```python
from build123d import *

# Parameters (mm, degrees)
SKETCH1_W           = 53.98
SKETCH1_H           = 1.59
SKETCH1_W_2         = 6.35
BOSS_EXTRUDE1_DEPTH = 20.64
SKETCH1_3_W         = 53.98
SKETCH1_3_H         = 1.59
SKETCH1_3_H_2       = 18.25
SKETCH1_3_R         = 3.175
SKETCH1_3_W_2       = 6.35
SKETCH1_3_H_3       = 19.84
BOSS_EXTRUDE2_DEPTH = 1.59


with BuildPart() as part:
    # Sketch1 → Boss-Extrude1 (new body)
    with BuildSketch(Plane(origin=(0, 0, 0), x_dir=(1, 0, 0), z_dir=(0, 1, 0))):
        with Locations((0, 0.005)):
            Rectangle(SKETCH1_W, SKETCH1_H)
        with Locations((-30.165, 0.005)):
            Rectangle(SKETCH1_W_2, SKETCH1_H)
        with Locations((30.165, 0.005)):
            Rectangle(SKETCH1_W_2, SKETCH1_H)
    extrude(amount=BOSS_EXTRUDE1_DEPTH)

    # Sketch1_3 → Boss-Extrude2 (add)
    # profile 1 of 4: a face of its own
    with BuildSketch(Plane(origin=(0, 0, 0), x_dir=(1, 0, 0), z_dir=(0, 1, 0))):
        with Locations((0, 0.005)):
            Rectangle(SKETCH1_3_W, SKETCH1_3_H)
    # profile 2 of 4: a face of its own
    with BuildSketch(Plane(origin=(0, 0, 0), x_dir=(1, 0, 0), z_dir=(0, 1, 0))):
        with Locations((0, 9.925)):
            Rectangle(SKETCH1_3_W, SKETCH1_3_H_2)
        with Locations(Location((-13.825, 10.08, 0), (0, 0, 90))):
            Circle(SKETCH1_3_R, mode=Mode.SUBTRACT)
        with Locations(Location((13.825, 10.08, 0), (0, 0, 90))):
            Circle(SKETCH1_3_R, mode=Mode.SUBTRACT)
    # profile 3 of 4: a face of its own
    with BuildSketch(Plane(origin=(0, 0, 0), x_dir=(1, 0, 0), z_dir=(0, 1, 0))):
        with Locations((-30.165, 9.13)):
            Rectangle(SKETCH1_3_W_2, SKETCH1_3_H_3)
    # profile 4 of 4: a face of its own
    with BuildSketch(Plane(origin=(0, 0, 0), x_dir=(1, 0, 0), z_dir=(0, 1, 0))):
        with Locations((30.165, 9.13)):
            Rectangle(SKETCH1_3_W_2, SKETCH1_3_H_3)
    extrude(amount=BOSS_EXTRUDE2_DEPTH)


solid = part.part
```
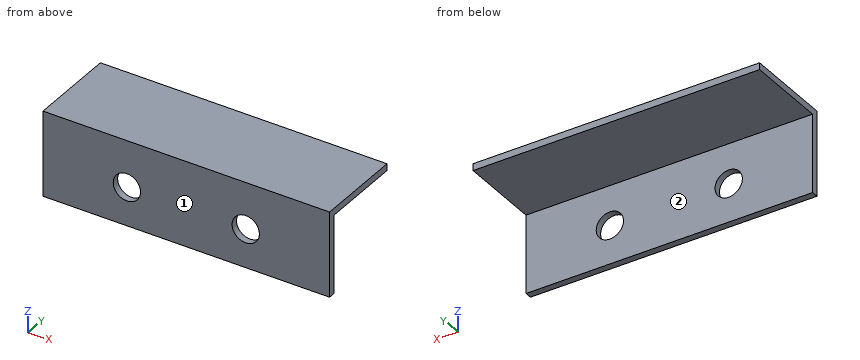
Can you work these out from the model? Positions are in its coordinate system, mm. Face numbers are marked on the shaded views. A direction names the side the tool comes from. Coordinates: 2 decimals unless noted, no trailing zeros. Write each loop counter-clockwise with the first axis right and the second up, starting at its lowest first coordinate (ties: lowest second). Pieces come first, ordered by that corner, then holes. Notation, with made-up numbers: M 56,-1.5 L 90,-1.5 A22 ccw 90,14.5 Z; hole C -14.75,71 d9. An arc over 180 degrees is marked long. Write item = value, one per line. Start each with the question number.
Q1. If we section it at B-B, the plane x = 24: Write out the boundary of the cut face in (y, z).
Q2. If we section it at C-C, the plane z = -16.75: Write out the boundary of the cut face in (x, y).
Q3. I'm going to push flat-ended pins straight in: pin 1 (4 mm diameter, centred on x = -2.5, y = 16, fed in from -Z); pin 2 (5 mm diameter, centred on x = 16.5, z = -4.5, fed in from +Y); pin 3 (4 mm diameter, centred on x = 13.825, z = -10.08, fed in from -Y). Where does each tip first touch, or does it pass through?
Q4. If we section it at D-D, the plane y = 2.5: Write out the boundary of the cut face in (x, z), then the cut area to 3 significant figures.
Q5. If I drill on L1, parallel to X at y = 0.3, z = -10.08; L2, parallel to Y at x = 24, z = -14.75; L3, parallel to Z at x = 28.5, y = 5, over which ranges is the centre line in solid material (lowest first)? Write a range as [from, to].
Q6. If we section it at A-A, the plane z = -10.08: Write out the boundary of the cut face in (x, y).
Q7. On a 3-axis mill with a long thin cutter (end or side, diameter ignored), from which of +Z, -Z, +X, -X, +Y, -Y can I reach the whole of each face in a straight line? I mean the marked faces 1 and 2. Say none if no direction works.
Check sheet entries:
q1.outline = M 0,-19.05 L 1.59,-19.05 L 1.59,-0.8 L 20.64,-0.8 L 20.64,0.79 L 0,0.79 Z
q2.outline = M -33.34,0 L 33.34,0 L 33.34,1.59 L -33.34,1.59 Z
q3.pin_1 = -0.8
q3.pin_2 = 1.59
q3.pin_3 = through
q4.outline = M -33.34,-0.8 L 33.34,-0.8 L 33.34,0.79 L -33.34,0.79 Z
q4.area = 106 mm²
q5.L1 = [-33.34, -17], [-10.65, 10.65], [17, 33.34]
q5.L2 = [0, 1.59]
q5.L3 = [-0.8, 0.79]
q6.outline = M -33.34,0 L -17,0 L -17,1.59 L -33.34,1.59 Z; M -10.65,0 L 10.65,0 L 10.65,1.59 L -10.65,1.59 Z; M 17,0 L 33.34,0 L 33.34,1.59 L 17,1.59 Z
q7.face_1 = +Z, -Z, +X, -X, -Y
q7.face_2 = -Z, +X, -X, +Y
